from build123d import *

# Parameters (mm, degrees)
F1_DEPTH      = 80
F0_W          = 2.5
F0_H          = 16
F0_W_2        = 6.5
F2_DEPTH      = 2.5
F3_SIZE       = 2
F4_R          = 3
F5_T1_DEPTH   = 87.5
F5_T3_DEPTH   = 16
F5_T8_DEPTH   = 16
F7_W          = 40
F7_H          = 60
F8_DEPTH      = 15
F6_R          = 4.65
F9_DEPTH      = 14
F9_DEPTH_BACK = 25
F10_R         = 4.65
F11_DEPTH     = 25


# Not quite as in the source:
# - a fillet or chamfer that OpenCascade refuses, or shapes differently, is made with other operations: its cross-section is extruded or revolved along the edge and cut away or added


with BuildPart() as f1:
    # F0 (on Top) → F1 (new body)
    with BuildSketch(Plane.XY):
        Polygon((-11.9039647728, 18.5), (-24.4039647728, 18.5), (-24.4039647728, -2.5), (49.5960352272, -2.5), (49.5960352272, 18.5), (37.0960352272, 18.5), (37.0960352272, 16), (44.5960352272, 16), (47.0960352272, 16), (47.0960352272, 0), (44.5960352272, 0), (-15.4039647728, 0), (-21.9039647728, 0), (-21.9039647728, 16), (-15.4039647728, 16), (-11.9039647728, 16), align=None)
    extrude(amount=F1_DEPTH)

    # F0 (on Top) → F2 (join)
    with BuildSketch(Plane.XY):
        with Locations((45.8460352272, 8)):
            Rectangle(F0_W, F0_H)
        with Locations((-18.6539647728, 8)):
            Rectangle(F0_W_2, F0_H)
    extrude(amount=F2_DEPTH)

    # F3
    f3_edges = [f1.edges().sort_by_distance(p)[0] for p in [
        (47.096035, 0, 41.25),
        (47.096035, 16, 41.25),
        (-21.903965, 0, 41.25),
        (-21.903965, 16, 41.25),
    ]]
    chamfer(f3_edges, length=F3_SIZE)

    # F4
    f4_edges = [f1.edges().sort_by_distance(p)[0] for p in [
        (-24.403965, 18.5, 40),
        (-24.403965, -2.5, 40),
        (49.596035, -2.5, 40),
        (49.596035, 18.5, 40),
    ]]
    fillet(f4_edges, radius=F4_R)

    # F5: fillet of radius 1.5 on 8 edges, made by hand

    # F5_s2 → F5_t1 (cut)
    with BuildSketch(Plane.XY.offset(-3.75)):
        with BuildLine():
            ThreePointArc((-11.9039647728, 17.5), (-12.343304601, 16.4393398282), (-13.4039647728, 16))
            Line((-13.4039647728, 16), (-11.9039647728, 16))
            Line((-11.9039647728, 16), (-11.9039647728, 17.5))
        make_face()
        with BuildLine():
            ThreePointArc((-13.4039647728, 18.5), (-12.343304601, 18.0606601718), (-11.9039647728, 17))
            Line((-11.9039647728, 17), (-11.9039647728, 18.5))
            Line((-11.9039647728, 18.5), (-13.4039647728, 18.5))
        make_face()
        with BuildLine():
            ThreePointArc((38.5960352272, 18.5), (37.5353750554, 18.0606601718), (37.0960352272, 17))
            Line((37.0960352272, 17), (37.0960352272, 18.5))
            Line((37.0960352272, 18.5), (38.5960352272, 18.5))
        make_face()
        with BuildLine():
            ThreePointArc((37.0960352272, 17.5), (37.5353750554, 16.4393398282), (38.5960352272, 16))
            Line((38.5960352272, 16), (37.0960352272, 16))
            Line((37.0960352272, 16), (37.0960352272, 17.5))
        make_face()
    extrude(amount=F5_T1_DEPTH, mode=Mode.SUBTRACT)

    # F5_s4 → F5_t3 (cut)
    with BuildSketch(Plane.XZ.offset(-16)):
        with BuildLine():
            ThreePointArc((46.0960352272, 0), (45.0353750554, 0.4393398282), (44.5960352272, 1.5))
            Line((44.5960352272, 1.5), (44.5960352272, 0))
            Line((44.5960352272, 0), (46.0960352272, 0))
        make_face()
        with BuildLine():
            ThreePointArc((-15.4039647728, 1), (-15.843304601, 2.0606601718), (-16.9039647728, 2.5))
            Line((-16.9039647728, 2.5), (-15.4039647728, 2.5))
            Line((-15.4039647728, 2.5), (-15.4039647728, 1))
        make_face()
        with BuildLine():
            ThreePointArc((-16.9039647728, 0), (-15.843304601, 0.4393398282), (-15.4039647728, 1.5))
            Line((-15.4039647728, 1.5), (-15.4039647728, 0))
            Line((-15.4039647728, 0), (-16.9039647728, 0))
        make_face()
    extrude(amount=F5_T3_DEPTH, mode=Mode.SUBTRACT)


with BuildPart() as f5_tool6:
    # F5_s7 → F5_t8 (new body)
    with BuildSketch(Plane.XZ.offset(-16)):
        with BuildLine():
            ThreePointArc((46.0960352272, 2.5), (45.0353750554, 2.0606601718), (44.5960352272, 1))
            Line((44.5960352272, 1), (44.5960352272, 2.5))
            Line((44.5960352272, 2.5), (46.0960352272, 2.5))
        make_face()
    extrude(amount=F5_T8_DEPTH)

    split(bisect_by=Plane(origin=(30.5480176136, 30.5480176136, 0), x_dir=(0, 0, 1), z_dir=(-0.7071067812, -0.7071067812, 0)), keep=Keep.TOP)

    split(bisect_by=Plane(origin=(22.5480176136, -22.5480176136, 0), x_dir=(0, 0, 1), z_dir=(-0.7071067812, 0.7071067812, 0)), keep=Keep.TOP)


with BuildPart() as f1_1:
    add(f1.part)

    # F5_t5: cut F5_tool6
    add(f5_tool6.part, mode=Mode.SUBTRACT)

    # F7 (on face) → F8 (join)
    with BuildSketch(Plane.XZ.offset(2.5)):
        with Locations((12.5960352272, 50)):
            Rectangle(F7_W, F7_H)
    extrude(amount=F8_DEPTH)

    # F6 (on face) → F9 (cut, two sides)
    with BuildSketch(Plane.XZ.offset(2.5)) as f9_sk:
        Polygon((20.8232765631, 44.1168472171), (16.7096558952, 51.2418472171), (8.4824145592, 51.2418472171), (4.3687938912, 44.1168472171), (8.4824145592, 36.9918472171), (16.7096558952, 36.9918472171), align=None)
        with Locations((12.5960352272, 44.1168472171)):
            Circle(F6_R, mode=Mode.SUBTRACT)
    extrude(amount=F9_DEPTH, mode=Mode.SUBTRACT)
    extrude(f9_sk.sketch, amount=-F9_DEPTH_BACK, mode=Mode.SUBTRACT)

    # F10 (on face) → F11 (cut)
    with BuildSketch(Plane(origin=(0, 0, 0), x_dir=(-1, 0, 0), z_dir=(0, 1, 0))):
        with Locations((-12.5960352272, 44.1168472171)):
            Circle(F10_R)
    extrude(amount=-F11_DEPTH, mode=Mode.SUBTRACT)


solid = f1_1.part
Part model, mm, in its own coordinate system. A direction names the side the tool comes from. Give positions to 0.01 mm unless a question says otherwise; leave off trailing zeros. Loops run counter-clockwise (first coordinate to the right, second up) from the corner with the lowest first, then second, coordinate; pieces in that order, holes last. Notation, with made-up numbers: (69, -30.75) -> (119, -30.75) arc R20 cw to (119, -7.75) -> close; hole circle Ø11 at (33.25, 52.25). An arc over 180 degrees is marked (long way). Write each question's results on one line, items separated by ' | '. Start each with the question number.
Q1. Band-saw the part on C-C on z = 9.5. List the corners of the cut face in (x, y), plus the area to 3 significant figures.
Q2. Pin check, flat tips, straight feed: P1, Ø7.5, axis at y = -10, z = 60.5, coming from the +X side; P2, Ø12, axis at x = 30, z = 39.5, coming from the +Y side; P3, Ø12, axis at x = 6, y = -9, coming from the -Z side. Stop position of each tip, or through.
Q3. Band-saw the part on A-A on x = 40.5. List the corners of the cut face in (y, z), plus the area to 3 significant figures.
Q4. Band-saw the part on B-B on y = 8.5. List the corners of the cut face in (x, z).
Q5. Band-saw the part on D-D on y = -13. List the corners of the cut face in (x, z), plus the area to 3 significant figures.
Q6. Which spindle directions (+Z, -Z, +X, -X, +Y, -Y) get a long thin tool onto all of the face, cutting with end or side? Do faces 5 (the face through (32.596, -10, 50)), 6 (the face through (-20.89, 15.014, 40.708)), 7 (the face through (12, -10, 20)), 8 (the face through (-7.404, -10, 50)). Say none if no direction does.
Q7. Pull direction Z, two halves, no side cores. Call faces 1 (the face through (-19, 8, 2.5)), 2 (the face through (6.454, -8.366, 47.729)), 3 (the face through (46.11, 14.986, 40.514)), 4 (the face through (6.4, -8.4, 40.6)): +Z half, -Z half, draft (parallel to the pull), parting line (faces both ways), or undercut.
Q8. Wall check: L1, parallel to X at y = 7.5, z = 60; L2, parallel to Y at x = 45, z = 31.5; L3, parallel to Z at x = -17, y = 5.5. Give the ranges that are in metal, low to high.
Results are:
1) outline: (-24.4, 0.5) arc R3 ccw to (-21.4, -2.5) -> (46.6, -2.5) arc R3 ccw to (49.6, 0.5) -> (49.6, 15.5) arc R3 ccw to (46.6, 18.5) -> (38.6, 18.5) arc R1.5 ccw to (37.12, 17.25) arc R1.5 ccw to (38.6, 16) -> (45.1, 16) -> (47.1, 14) -> (47.1, 2) -> (45.1, 0) -> (-19.9, 0) -> (-21.9, 2) -> (-21.9, 14) -> (-19.9, 16) -> (-13.4, 16) arc R1.5 ccw to (-11.92, 17.25) arc R1.5 ccw to (-13.4, 18.5) -> (-21.4, 18.5) arc R3 ccw to (-24.4, 15.5) -> close | area: 326 mm²
2) P1: stops at x = 32.6 | P2: stops at y = 0 | P3: stops at z = 20
3) outline: (-2.5, 0) -> (0, 0) -> (0, 80) -> (-2.5, 80) -> close; (16, 0) -> (18.5, 0) -> (18.5, 80) -> (16, 80) -> close | area: 400 mm²
4) outline: (-24.4, 0) -> (-16.9, 0) arc R1.5 ccw to (-15.42, 1.25) arc R1.5 ccw to (-16.9, 2.5) -> (-21.9, 2.5) -> (-21.9, 80) -> (-24.4, 80) -> close; (44.62, 1.25) arc R1.5 ccw to (46.1, 0) -> (49.6, 0) -> (49.6, 80) -> (47.1, 80) -> (47.1, 2.5) -> (46.1, 2.5) arc R1.5 ccw to start
5) outline: (-7.4, 20) -> (32.6, 20) -> (32.6, 80) -> (-7.4, 80) -> close; hole (4.37, 44.12) -> (8.48, 36.99) -> (16.71, 36.99) -> (20.82, 44.12) -> (16.71, 51.24) -> (8.48, 51.24) -> close | area: 2,220 mm²
6) face 5: +Z, -Z, +X, -Y | face 6: +Z | face 7: -Z, +X, -X, -Y | face 8: +Z, -Z, -X, -Y
7) face 1: +Z half | face 2: undercut | face 3: draft | face 4: undercut
8) L1: x = -24.4 to -21.9, 47.1 to 49.6 | L2: y = -2.5 to 0, 16 to 18.5 | L3: z = 0 to 2.5
